CAD build for the part. Positions are in the model's coordinates, mm. A direction names the side the tool comes from. Give positions to 0.01 mm unless a question says otherwise; leave off trailing zeros. Order: outer loops, then holes, each group sorted by start corner. A loop starts at its lowest first (then second) coordinate and runs counter-clockwise, first axis right, second up.
Item 1: Wall check: L1, parallel to X at y = 5, z = 32; L2, parallel to Y at x = -12, z = 13; L3, parallel to Z at x = 16.5, y = 22. Give the ranges that are in metal, low to high.
Item 2: Two-plate mould, pull along Z, no slides. Class faces 4 (the flat face through (0, -27, 37.8)), 5 (the flat face through (0, 27, 41.6)), 6 (the flat face through (18, -27, 37.8)), 7 (the flat face through (26, -11.5, 40)): released by +Z, released by -Z, zero draft, split by the parting line, or undercut.
Item 3: Band-saw the part on B-B on z = 29. Count the separate pieces of the cut face and the enclosed holes in it, plus the area to 3 significant figures.
Item 4: Flat gauge pins, fed straight in: P1, Ø3, axis at x = -15, y = -19, coming from the +Z side; P2, Ø0.8, axis at y = 27.5, z = 36, coming from the +X side; P3, Ø4, axis at y = -21, z = 36, coming from the -X side. Where does each tip first touch, or does it go through?
Item 5: Band-saw the part on D-D on x = -10. Give the cut face in (y, z), plus the area to 3 significant figures.
Item 6: Band-saw the part on A-A on y = 6.5. Give the cut face in (x, z).
Item 7: Band-saw the part on C-C on z = 15.5. Give the cut face in (x, y).
Item 8: Which spindle directions (+Z, -Z, +X, -X, +Y, -Y) get a long thin tool onto all of the face, cutting with end or side? Do faces 1 (the flat face through (23.5, 27, 34)), 2 (the flat face through (-26, 16, 37.8)), 3 (the flat face through (-3.1, 27, 36)). Say none if no direction does.
```python
from build123d import *

# Parameters (mm, degrees)
SKETCH041_W          = 58.2
SKETCH041_H          = 55.7
PAD012_DEPTH         = 1.6
SKETCH046_W          = 53.7
SKETCH046_H          = 55.7
SKETCH046_W_2        = 50.5
SKETCH046_H_2        = 52.5
PAD014_DEPTH         = 40
FILLET005_R          = 1
SKETCH039_W          = 6.2
SKETCH039_H          = 4
SKETCH039_W_2        = 5
POCKET011_DEPTH      = 27.851
POCKET011_DEPTH_BACK = 27.851
SKETCH040_W          = 9
SKETCH040_H          = 3.8
POCKET013_DEPTH      = 31.351
POCKET013_DEPTH_BACK = 26.851
SKETCH042_R          = 3.2
PAD013_DEPTH         = 3
SKETCH045_R          = 1.75
POCKET012_DEPTH      = 4.601


with BuildPart() as part:
    # Sketch041 → Pad012 (new body)
    with BuildSketch(Plane.XY):
        with Locations((-2.25, 0)):
            Rectangle(SKETCH041_W, SKETCH041_H)
    extrude(amount=PAD012_DEPTH)

    # Sketch046 → Pad014 (join)
    with BuildSketch(Plane.XY.offset(1.6)):
        Rectangle(SKETCH046_W, SKETCH046_H)
        Rectangle(SKETCH046_W_2, SKETCH046_H_2, mode=Mode.SUBTRACT)
    extrude(amount=PAD014_DEPTH)

    # Fillet005
    fillet005_edges = [part.edges().sort_by_distance(p)[0] for p in [
        (-31.35, -27.85, 0.8),
        (-31.35, 27.85, 0.8),
        (-26.85, 27.85, 21.6),
        (-26.85, -27.85, 21.6),
        (26.85, -27.85, 20.8),
        (25.25, 26.25, 21.6),
        (-25.25, 26.25, 21.6),
        (26.85, 27.85, 20.8),
        (-25.25, -26.25, 21.6),
        (25.25, -26.25, 21.6),
        (0, 26.25, 1.6),
        (-25.25, 0, 1.6),
        (0, -26.25, 1.6),
        (25.25, 0, 1.6),
    ]]
    fillet(fillet005_edges, radius=FILLET005_R)

    # Sketch039 → Pocket011 (cut, two sides)
    with BuildSketch(Plane.XZ) as pocket011_sk:
        with Locations((0, 35.8)):
            Rectangle(SKETCH039_W, SKETCH039_H)
        with Locations((-18, 35.8)):
            Rectangle(SKETCH039_W_2, SKETCH039_H)
        with Locations((18, 35.8)):
            Rectangle(SKETCH039_W_2, SKETCH039_H)
        with BuildLine():
            Line((22.5, 41.6), (23.5, 41.6))
            Line((23.5, 41.6), (23.5, 26.6))
            ThreePointArc((22.5, 27.6), (22.792893, 26.892893), (23.5, 26.6))
            Line((22.5, 27.6), (22.5, 41.6))
        make_face()
        with BuildLine():
            Line((-23.5, 41.6), (-22.5, 41.6))
            Line((-22.5, 41.6), (-22.5, 27.6))
            ThreePointArc((-23.5, 26.6), (-22.792893, 26.892893), (-22.5, 27.6))
            Line((-23.5, 26.6), (-23.5, 41.6))
        make_face()
    extrude(amount=-POCKET011_DEPTH, mode=Mode.SUBTRACT)
    extrude(pocket011_sk.sketch, amount=POCKET011_DEPTH_BACK, mode=Mode.SUBTRACT)

    # Sketch040 → Pocket013 (cut, two sides)
    with BuildSketch(Plane.YZ) as pocket013_sk:
        with Locations((-16, 39.7)):
            Rectangle(SKETCH040_W, SKETCH040_H)
        with Locations((16, 39.7)):
            Rectangle(SKETCH040_W, SKETCH040_H)
        with BuildLine():
            Line((-18.733, 22.8), (18.733, 22.8))
            ThreePointArc((23.733, 17.8), (22.268534, 21.335534), (18.733, 22.8))
            Line((23.733, 1.6), (23.733, 17.8))
            Line((-23.733, 1.6), (23.733, 1.6))
            Line((-23.733, 17.8), (-23.733, 1.6))
            ThreePointArc((-18.733, 22.8), (-22.268534, 21.335534), (-23.733, 17.8))
        make_face()
    extrude(amount=-POCKET013_DEPTH, mode=Mode.SUBTRACT)
    extrude(pocket013_sk.sketch, amount=POCKET013_DEPTH_BACK, mode=Mode.SUBTRACT)

    # Sketch042 → Pad013 (join)
    with BuildSketch(Plane.XY.offset(1.6)):
        with Locations((-15.348, 15.621)):
            Circle(SKETCH042_R)
        with Locations((-28.048, -19.431)):
            Circle(SKETCH042_R)
        with Locations((-15.348, -19.431)):
            Circle(SKETCH042_R)
        with Locations((-28.048, 15.621)):
            Circle(SKETCH042_R)
    extrude(amount=PAD013_DEPTH)

    # Sketch045 → Pocket012 (cut, through all)
    with BuildSketch(Plane.XY.offset(4.6)):
        with Locations((-28.048, 15.621)):
            Circle(SKETCH045_R)
        with Locations((-15.348, 15.621)):
            Circle(SKETCH045_R)
        with Locations((-15.348, -19.431)):
            Circle(SKETCH045_R)
        with Locations((-28.048, -19.431)):
            Circle(SKETCH045_R)
    extrude(amount=-POCKET012_DEPTH, mode=Mode.SUBTRACT)


solid = part.part
```
The answers:
1. L1: x = -26.85 to -25.25, 25.25 to 26.85
1. L2: y = -27.85 to -26.25, 26.25 to 27.85
1. L3: z = 0 to 1.6
2. face 4: undercut
2. face 5: released by +Z
2. face 6: undercut
2. face 7: zero draft
3. separate pieces: 4
3. enclosed holes: 0
3. area: 333 mm2
4. P1: stops at z = 4.6
4. P2: stops at x = 26.82
4. P3: stops at x = -26.85
5. outline: (-27.85, 0) - (27.85, 0) - (27.85, 41.6) - (26.25, 41.6) - (26.25, 2.6) arc R1 cw to (25.25, 1.6) - (-25.25, 1.6) arc R1 cw to (-26.25, 2.6) - (-26.25, 41.6) - (-27.85, 41.6) - close
5. area: 218 mm2
6. outline: (-31.35, 0) - (26.85, 0) - (26.85, 1.6) - (-31.35, 1.6) - close; (-26.85, 22.8) - (-25.25, 22.8) - (-25.25, 41.6) - (-26.85, 41.6) - close; (25.25, 22.8) - (26.85, 22.8) - (26.85, 41.6) - (25.25, 41.6) - close
7. outline: (-26.85, -26.85) arc R1 ccw to (-25.85, -27.85) - (25.85, -27.85) arc R1 ccw to (26.85, -26.85) - (26.85, -23.73) - (25.25, -23.73) - (25.25, -25.25) arc R1 cw to (24.25, -26.25) - (-24.25, -26.25) arc R1 cw to (-25.25, -25.25) - (-25.25, -23.73) - (-26.85, -23.73) - close; (-26.85, 23.73) - (-25.25, 23.73) - (-25.25, 25.25) arc R1 cw to (-24.25, 26.25) - (24.25, 26.25) arc R1 cw to (25.25, 25.25) - (25.25, 23.73) - (26.85, 23.73) - (26.85, 26.85) arc R1 ccw to (25.85, 27.85) - (-25.85, 27.85) arc R1 ccw to (-26.85, 26.85) - close
8. face 1: +Z, +Y, -Y
8. face 2: +Z, +X, -X
8. face 3: +Y, -Y
